Autodesk Inventor part; units mm, degrees
ref_plane "YZ Plane" through (0, 0, 0) normal (1, 0, 0) x (0, 1, 0)
ref_plane "XZ Plane" through (0, 0, 0) normal (0, 1, 0) x (-1, 0, 0)
ref_plane "XY Plane" through (0, 0, 0) normal (0, 0, 1) x (1, 0, 0)
sketch "Sketch1" plane through (0, 0, 0) normal (0, 0, 1) x (1, 0, 0)
  line L0 (-14.2785, 0) -> (14.2785, 0) construction
  line L1 (-14.2785, -4) -> (14.2785, -4)
  line L2 (14.2785, 4) -> (-14.2785, 4)
  arc A0 (-14.2785, 4) -> (-14.2785, -4) centre (-14.2785, 0) ccw
  arc A1 (14.2785, -4) -> (14.2785, 4) centre (14.2785, 0) ccw
  circle A2 centre (-14.2785, 0) radius 1.75
  circle A3 centre (14.2785, 0) radius 1.75
  point P0 (0, 0)
  dimension "d0" = 4
  dimension "d1" = 3.5
  dimension "d2" = 3.5
  dimension "d3" = 28.557
extrude "Extrusion1" add sketch "Sketch1" along normal blind 4
sketch "Sketch2" plane through (0, 0, 4) normal (0, 0, 1) x (1, 0, 0)
  circle A0 centre (14.2785, 0) radius 1.75
  circle A1 centre (14.2785, 0) radius 3
  point P0 (0, 0)
  dimension "d6" = 6
extrude "Extrusion2" cut sketch "Sketch2" against normal blind 2
properties part number "mechanism_2"
Here's how the part is built. I have some questions about the finished solid (model axes, mm). A direction names the side the tool comes from. Round coordinates to 2 decimals unless told otherwise and drop trailing zeros. Loops run counter-clockwise (first coordinate to the right, second up) from the corner with the lowest first, then second, coordinate; pieces in that order, holes last. Notation, with made-up numbers: M 83.5,32.5 L 110.5,32.5 A30 cw 110.5,70.5 Z; hole C 16.5,-10.75 d5. An arc over 180 degrees is marked long. Write each question's results on one line, items separated by ' | '. Start each with the question number.
(1) Will these pins go through, and if not, where does the flat tip stop? P1, Ø4.5, axis at x = -14.28, y = 0, coming from the -Z side; P2, Ø2, axis at y = -2.5, z = 1, coming from the -X side.
(2) I want a section at C-C (z = 1.05). Please give me the cut outline in (x, y), then the cut area to 3 significant figures.
(3) Thinking about a two-plate mould opening in X: for faces 1 (the cylindrical face through (-18.278, -0.088, 1.972)), 2 (the flat face through (0, 4, 2)), 3 (the flat face through (16, -1, 2)), 4 (the cylindrical face through (18.278, 0.088, 1.972)), which applies, pulls with the +X half, pulls with the -X half, needs draft (parallel to the pull), parting line crosses it, or undercut?
(4) I want a section at D-D (y = 3.5). Please give me the cut outline in (x, z) (3 decimals), then the cut area to 3 significant figures.
(5) I want a section at A-A (y = 0). Please give me the cut outline in (x, z), then the cut area to 3 significant figures.
(6) I want a section at B-B (z = 2.7). Please give me the cut outline in (x, y).
(7) If I drill on probe 1 along X at (y, z) = (0.25, 2.05); probe 2 along Z at (x, y) = (13, -2.5); probe 3 along X at (y, z) = (-2.5, 1.3), over which ranges is the centre line in solid material (lowest first)? Write a range as from..to.
(8) On a 3-axis mill with a long thin cutter (end or side, diameter ignored), from which of +Z, -Z, +X, -X, +Y, -Y can I reach the whole of each face in a straight line? I mean faces 5 (the cylindrical face through (12.53, -0.08, 0.99)), 6 (the cylindrical face through (11.28, 0.13, 3.01)). Say none if no direction works.
Solved:
1) P1: stops at z = 0 | P2: stops at x = -17.99
2) outline: M -14.28,-4 L 14.28,-4 A4 ccw 14.28,4 L -14.28,4 A4 ccw Z; hole C -14.28,0 d3.5; hole C 14.28,0 d3.5 | area: 259 mm²
3) face 1: pulls with the -X half | face 2: needs draft | face 3: undercut | face 4: pulls with the +X half
4) outline: M -16.215,0 L 16.215,0 L 16.215,4 L -16.215,4 Z | area: 130 mm²
5) outline: M -18.28,0 L -16.03,0 L -16.03,4 L -18.28,4 Z; M -12.53,0 L 12.53,0 L 12.53,2 L 11.28,2 L 11.28,4 L -12.53,4 Z; M 16.03,0 L 18.28,0 L 18.28,4 L 17.28,4 L 17.28,2 L 16.03,2 Z | area: 113 mm²
6) outline: M -14.28,-4 L 14.28,-4 A4 ccw 14.28,4 L -14.28,4 A4 ccw Z; hole C -14.28,0 d3.5; hole C 14.28,0 d6
7) probe 1: x = -18.27..-16.01, -12.55..11.29, 17.27..18.27 | probe 2: z = 0..2 | probe 3: x = -17.4..17.4
8) face 5: +Z, -Z | face 6: +Z
